The listing builds one solid part. Answer for the finished solid, in the listing's coordinates (mm). Round coordinates to 2 decimals unless told otherwise and drop trailing zeros. Write each loop counter-clockwise with the first axis right and the second up, starting at its lowest first coordinate (ties: lowest second). Pieces come first, ordered by that corner, then holes.
(1) Find the intervals of material crossed by probe 1 along Y at (x, z) = (71, 24.9); probe 2 along X at (y, z) = (30, 24.85); probe 3 along X at (y, z) = (29, 24.9), in increasing order.
(2) This flat-tipped pin is pushed along its axis until it touches: pin 1 Ø3 at (x, y) = (-71, -42.5) entering from -Z. Where does it stop, or does it pass through?
(3) A cutting plane is placed at B-B, the plane z = 24.8. Give the number of separate pieces and of enclosed holes in the cut face, and give its area (3 significant figures).
(4) A cutting plane is placed at C-C, the plane x = -22.5. Give the vertices of the cut face in (y, z), and give its area (3 significant figures).
(5) A cutting plane is placed at A-A, the plane x = 71. Give the vertices of the cut face in (y, z).
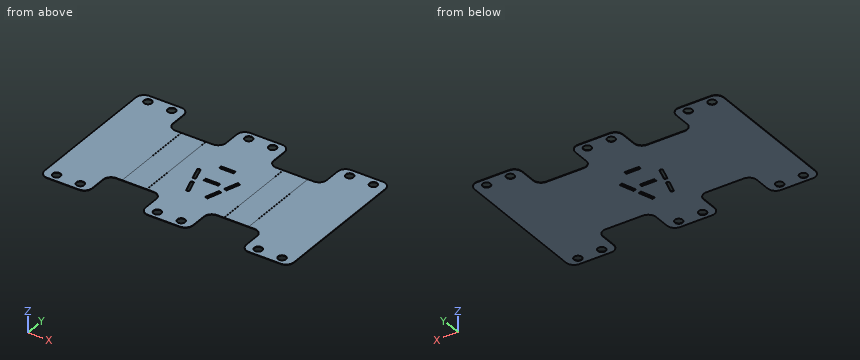
from build123d import *

# Parameters (mm, degrees)
F0_R     = 2.5
F1_DEPTH = 25
F2_DEPTH = 25
F3_W     = 9.2
F3_H     = 1.9
F4_DEPTH = 25
F5_R     = 5
F7_DEPTH = 40
F8_W     = 165.974393075
F8_H     = 32.5776245729
F9_DEPTH = 97


with BuildPart() as f1:
    # F0 (on Top) → F1 (new body)
    with BuildSketch(Plane.XY):
        Polygon((15, 47.5), (-15, 47.5), (-15, 27.5), (-48.5, 27.5), (-48.5, 47.5), (-78.5, 47.5), (-78.5, -47.5), (-48.5, -47.5), (-48.5, -27.5), (-15, -27.5), (-15, -47.5), (15, -47.5), (15, -27.5), (48.5, -27.5), (48.5, -47.5), (78.5, -47.5), (78.5, 47.5), (48.5, 47.5), (48.5, 27.5), (15, 27.5), align=None)
        with Locations((-71, -42.5)):
            Circle(F0_R, mode=Mode.SUBTRACT)
        with Locations((-56, -42.5)):
            Circle(F0_R, mode=Mode.SUBTRACT)
        with Locations((-7.5, -42.5)):
            Circle(F0_R, mode=Mode.SUBTRACT)
        with Locations((7.5, -42.5)):
            Circle(F0_R, mode=Mode.SUBTRACT)
        with Locations((56, -42.5)):
            Circle(F0_R, mode=Mode.SUBTRACT)
        with Locations((71, -42.5)):
            Circle(F0_R, mode=Mode.SUBTRACT)
        with Locations((-71, 42.5)):
            Circle(F0_R, mode=Mode.SUBTRACT)
        with Locations((-56, 42.5)):
            Circle(F0_R, mode=Mode.SUBTRACT)
        with Locations((-7.5, 42.5)):
            Circle(F0_R, mode=Mode.SUBTRACT)
        with Locations((7.5, 42.5)):
            Circle(F0_R, mode=Mode.SUBTRACT)
        with Locations((56, 42.5)):
            Circle(F0_R, mode=Mode.SUBTRACT)
        with Locations((71, 42.5)):
            Circle(F0_R, mode=Mode.SUBTRACT)
    extrude(amount=F1_DEPTH)

    # F0 (on Top) → F2 (cut)
    with BuildSketch(Plane.XY):
        Polygon((15, 47.5), (-15, 47.5), (-15, 27.5), (-48.5, 27.5), (-48.5, 47.5), (-78.5, 47.5), (-78.5, -47.5), (-48.5, -47.5), (-48.5, -27.5), (-15, -27.5), (-15, -47.5), (15, -47.5), (15, -27.5), (48.5, -27.5), (48.5, -47.5), (78.5, -47.5), (78.5, 47.5), (48.5, 47.5), (48.5, 27.5), (15, 27.5), align=None)
        with Locations((-71, -42.5)):
            Circle(F0_R, mode=Mode.SUBTRACT)
        with Locations((-56, -42.5)):
            Circle(F0_R, mode=Mode.SUBTRACT)
        with Locations((-7.5, -42.5)):
            Circle(F0_R, mode=Mode.SUBTRACT)
        with Locations((7.5, -42.5)):
            Circle(F0_R, mode=Mode.SUBTRACT)
        with Locations((56, -42.5)):
            Circle(F0_R, mode=Mode.SUBTRACT)
        with Locations((71, -42.5)):
            Circle(F0_R, mode=Mode.SUBTRACT)
        with Locations((-71, 42.5)):
            Circle(F0_R, mode=Mode.SUBTRACT)
        with Locations((-56, 42.5)):
            Circle(F0_R, mode=Mode.SUBTRACT)
        with Locations((-7.5, 42.5)):
            Circle(F0_R, mode=Mode.SUBTRACT)
        with Locations((7.5, 42.5)):
            Circle(F0_R, mode=Mode.SUBTRACT)
        with Locations((56, 42.5)):
            Circle(F0_R, mode=Mode.SUBTRACT)
        with Locations((71, 42.5)):
            Circle(F0_R, mode=Mode.SUBTRACT)
    extrude(amount=-F2_DEPTH, mode=Mode.SUBTRACT)

    # F3 (on face) → F4 (cut)
    with BuildSketch(Plane.XY.offset(25)):
        with Locations((0, 11.5)):
            Rectangle(F3_W, F3_H)
        with Locations((0, -2.8)):
            Rectangle(F3_W, F3_H)
        Polygon((-8.8533070383, -4.6304771843), (-11.71855, 4.11197), (-13.5240553968, 3.5202350405), (-10.658812435, -5.2222121438), align=None)
        Polygon((-6.7587246898, -17.1221841819), (-4.953219293, -16.5304492224), (-7.8184622548, -7.7880020381), (-9.6239676515, -8.3797369976), align=None)
        Polygon((13.5240553968, 3.5202350405), (11.71855, 4.11197), (8.8533070383, -4.6304771843), (10.658812435, -5.2222121438), align=None)
        Polygon((7.8184622548, -7.7880020381), (4.953219293, -16.5304492224), (6.7587246898, -17.1221841819), (9.6239676515, -8.3797369976), align=None)
    extrude(amount=-F4_DEPTH, mode=Mode.SUBTRACT)

    # F5
    f5_edges = [f1.edges().sort_by_distance(p)[0] for p in [
        (-48.5, 47.5, 12.5),
        (-48.5, 27.5, 12.5),
        (15, 47.5, 12.5),
        (15, 27.5, 12.5),
        (78.5, 47.5, 12.5),
        (48.5, 47.5, 12.5),
        (-15, 47.5, 12.5),
        (48.5, 27.5, 12.5),
        (-15, 27.5, 12.5),
        (-78.5, 47.5, 12.5),
        (15, -27.5, 12.5),
        (15, -47.5, 12.5),
        (78.5, -47.5, 12.5),
        (-48.5, -27.5, 12.5),
        (-48.5, -47.5, 12.5),
        (48.5, -27.5, 12.5),
        (48.5, -47.5, 12.5),
        (-15, -27.5, 12.5),
        (-15, -47.5, 12.5),
        (-78.5, -47.5, 12.5),
    ]]
    fillet(f5_edges, radius=F5_R)

    # F6 (on Front) → F7 (cut, symmetric)
    with BuildSketch(Plane.XZ):
        Polygon((-38.85, 32.4957541127), (-40.85, 32.4957541127), (-39.85, 24.9), align=None)
        Polygon((39.85, 24.9), (40.85, 32.4957541127), (38.85, 32.4957541127), align=None)
        Polygon((-23.35, 32.4957541127), (-25.35, 32.4957541127), (-24.35, 24.9), align=None)
        Polygon((24.35, 24.9), (25.35, 32.4957541127), (23.35, 32.4957541127), align=None)
    extrude(amount=F7_DEPTH, both=True, mode=Mode.SUBTRACT)

    # F8 (on face) → F9 (cut)
    with BuildSketch(Plane.XZ.offset(47.5)):
        with Locations((2.9871965375, 8.4111877136)):
            Rectangle(F8_W, F8_H)
    extrude(amount=-F9_DEPTH, mode=Mode.SUBTRACT)


solid = f1.part
Solutions:
1. probe 1: y = -47.5 to -45, -40 to 40, 45 to 47.5
1. probe 2: x = -78.5 to -47.83, -15.67 to 15.67, 47.83 to 78.5
1. probe 3: x = -78.5 to -47.07, -16.43 to 16.43, 47.07 to 78.5
2. pin 1: passes through
3. separate pieces: 1
3. enclosed holes: 18
3. area: 11,900 mm2
4. outline: (-27.5, 24.7) - (27.5, 24.7) - (27.5, 25) - (-27.5, 25) - close
4. area: 16.5 mm2
5. outline: (-47.5, 24.7) - (-45, 24.7) - (-45, 25) - (-47.5, 25) - close; (-40, 24.7) - (40, 24.7) - (40, 25) - (-40, 25) - close; (45, 24.7) - (47.5, 24.7) - (47.5, 25) - (45, 25) - close
